Check sheet for the drawn part. Datum: minimum x, y, z corner. Units: mm. A direction names the side the tool comes from. Round coordinates to 2 decimals unless told otherwise and drop trailing zeros. Write each loop counter-clockwise with the first axis right and the second up, starting at its lowest first coordinate (ties: lowest second). Pieces come first, ordered by that corner, then holes. Notation, with made-up numbers: (-1, -24) -> (24, -24) arc R22 cw to (24, 15) -> close; hole circle Ø2 at (50, 22.5). An arc over 180 degrees is marked (long way). One line per item, written item: value. Start each with the question number.
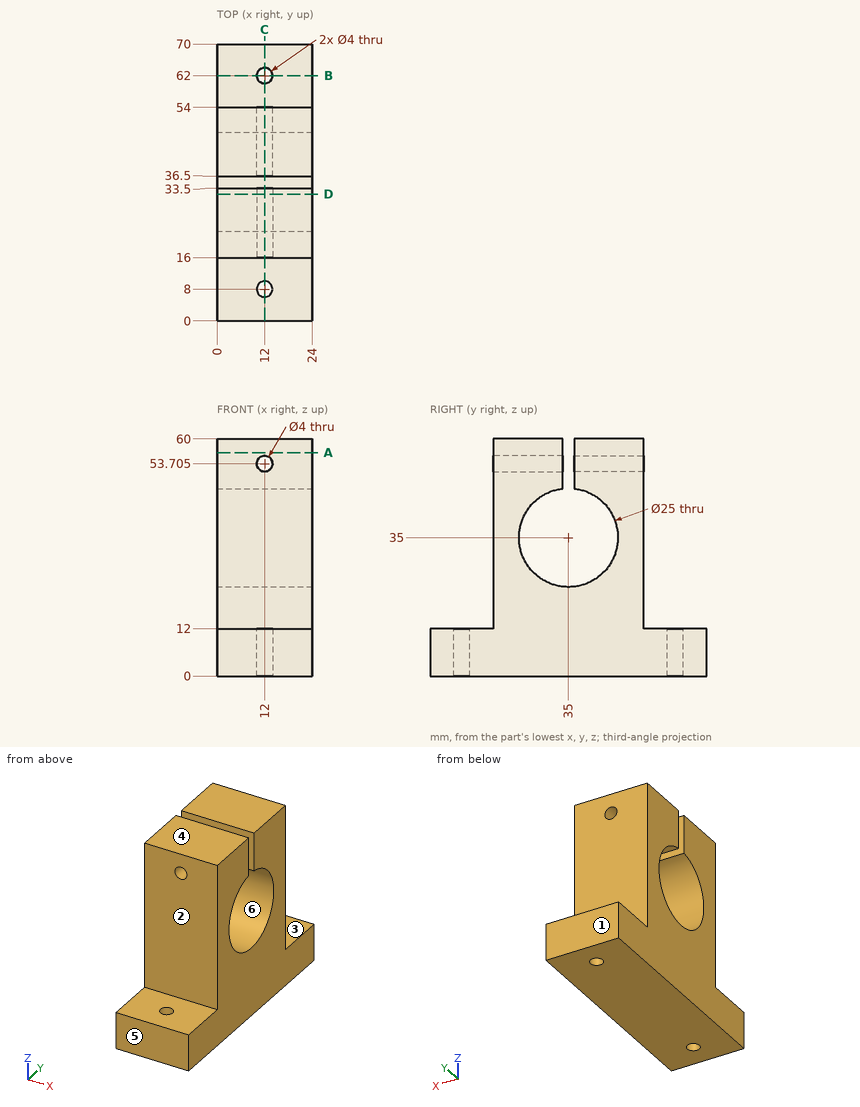
1. Cross-section at B-B (y = 62). Record the cut outline in (x, z), plus the area to 3 significant figures.
2. Depth check by flat-ended pin: pin 1 Ø12 at (x, z) = (13.5, 28.5) entering from +Y; pin 2 Ø14 at (x, z) = (7, 52) entering from -Y; pin 3 Ø3.5 at (x, z) = (12, 53.7) entering from +Y; pin 4 Ø5 at (x, y) = (15, 60) entering from +Z. Enter the tip coordinate at first touch or a pass-through.
3. Cross-section at A-A (z = 56.5). Record the cut outline in (x, y).
4. Material ranges on probe 1 along Y at (x, z) = (12, 6.75); probe 2 along Y at (x, z) = (8, 35.5); probe 3 along Z at (x, y) = (12, 42.5) (1 decimal), recorded low to high.
5. Release check for a two-part mould opening along Y. For the marked faces 4, 5 and 6 record: +Y half, -Y half, draft (parallel to the pull), parting line (faces both ways), or undercut.
6. Access from +Z, -Z, +X, -X, +Y, -Y to the whole of each face (thin tool, end or side, straight path). Record for the marked faces 1, 2 and 3.
7. Cross-section at D-D (y = 32). Record the cut outline in (x, z) (1 decimal), plus the area to 3 significant figures.
8. Cross-section at C-C (x = 12). Record the cut outline in (y, z) (1 decimal).
Working result:
1. outline: (0, 0) -> (10, 0) -> (10, 12) -> (0, 12) -> close; (14, 0) -> (24, 0) -> (24, 12) -> (14, 12) -> close
1. area: 240 mm^2
2. pin 1: stops at y = 54
2. pin 2: stops at y = 16
2. pin 3: passes through
2. pin 4: stops at z = 12
3. outline: (0, 16) -> (24, 16) -> (24, 33.5) -> (0, 33.5) -> close; (0, 36.5) -> (24, 36.5) -> (24, 54) -> (0, 54) -> close
4. probe 1: y = 0 to 6, 10 to 60, 64 to 70
4. probe 2: y = 16 to 22.51, 47.49 to 54
4. probe 3: z = 0 to 25, 45 to 51.7, 55.7 to 60
5. face 4: draft
5. face 5: -Y half
5. face 6: undercut
6. face 1: +Z, -Z, +X, -X, +Y
6. face 2: +Z, +X, -X, -Y
6. face 3: +Z, +X, -X, +Y
7. outline: (0, 0) -> (24, 0) -> (24, 22.9) -> (0, 22.9) -> close; (0, 47.1) -> (24, 47.1) -> (24, 60) -> (0, 60) -> close; hole circle Ø4 at (12, 53.7)
7. area: 845 mm^2
8. outline: (0, 0) -> (6, 0) -> (6, 12) -> (0, 12) -> close; (10, 0) -> (60, 0) -> (60, 12) -> (54, 12) -> (54, 51.7) -> (36.5, 51.7) -> (36.5, 47.4) arc R12.5 cw (long way) to (33.5, 47.4) -> (33.5, 51.7) -> (16, 51.7) -> (16, 12) -> (10, 12) -> close; (16, 55.7) -> (33.5, 55.7) -> (33.5, 60) -> (16, 60) -> close; (36.5, 55.7) -> (54, 55.7) -> (54, 60) -> (36.5, 60) -> close; (64, 0) -> (70, 0) -> (70, 12) -> (64, 12) -> close
